Source: CAD feature listing. Evaluate the final solid. Frame: model axes, mm. Face numbers are marked on the shaded views. Give positions to 0.01 mm unless a question says otherwise; leave off trailing zeros. Order: outer loops, then holes, each group sorted by start corner. A loop starts at its lowest first (then second) coordinate and runs counter-clockwise, first axis right, second up.
1) Material intervals for line 1 (Z direction, x = 18.25, y = 0.6); line 2 (Z direction, x = 18.25, y = 3.2); line 3 (X direction, y = 1, z = 38.5), sorted ascending.
2) Draft query along X for the marked faces 1, 2 and 3. Return one class per face: released by +X, released by -X, zero draft, split by the parting line, or undercut.
3) First-contact query: P1, Ø4, axis at y = 10.5, z = -13.5, coming from the +X side; P2, Ø10, axis at y = 13.5, z = 25, coming from the -X side; P3, Ø11, axis at x = 41, y = 6.5, coming from the -Z side. Flat tips, straight axial feed; report the tip coordinate or a pass-through.
4) Section C-C, the plane x = 18.25. Return loops of the section in (y, z).
5) Section D-D, the plane z = 16.5. Return loops of the section in (x, y), plus the area to 3 significant figures.
6) Section B-B, the plane x = 0. Return loops of the section in (y, z).
7) Section A-A, the plane z = 0. Return loops of the section in (x, y), plus the area to 3 significant figures.
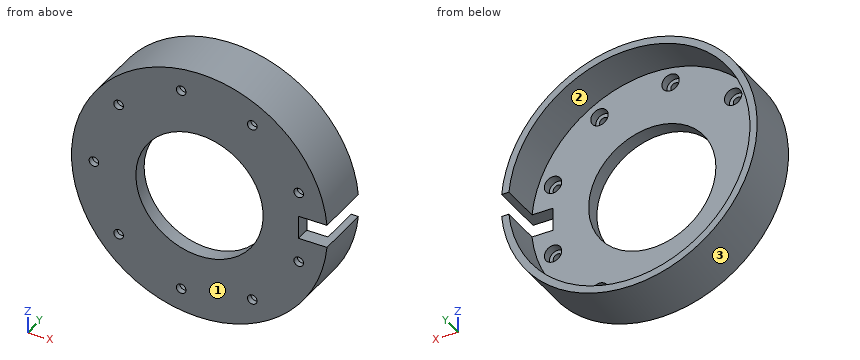
Autodesk Inventor part; units mm, degrees
ref_plane "YZ Plane" through (0, 0, 0) normal (1, 0, 0) x (0, 1, 0)
ref_plane "XZ Plane" through (0, 0, 0) normal (0, 1, 0) x (-1, 0, 0)
ref_plane "XY Plane" through (0, 0, 0) normal (0, 0, 1) x (1, 0, 0)
sketch "スケッチ1" plane through (0, 0, 0) normal (0, 1, 0) x (-1, 0, 0)
  circle A0 centre (0, 0) radius 44.25
  circle A1 centre (0, 0) radius 22
  dimension "d0" = 88.5
  dimension "d3" = 44
extrude "押し出し1" add sketch "スケッチ1" along normal blind 5
sketch "スケッチ2" plane through (0, 5, 0) normal (0, 1, 0) x (1, 0, 0)
  circle A0 centre (0, 0) radius 36.5
  point P0 (-36.5, 0)
  point P1 (-27.9606, -23.4617)
  point P2 (-6.3382, -35.9455)
  point P3 (18.25, -31.6099)
  point P4 (34.2988, -12.4837)
  point P5 (34.2988, 12.4837)
  point P6 (18.25, 31.6099)
  point P7 (-6.3382, 35.9455)
  point P8 (-27.9606, 23.4617)
  dimension "d4" = 73
  dimension "d7" = 360
hole "穴1" at (-36.5, 5, 0) at (-27.9606, 5, 23.4617) at (-6.3382, 5, 35.9455) at (18.25, 5, 31.6099) at (34.2988, 5, 12.4837) at (34.2988, 5, -12.4837) at (18.25, 5, -31.6099) at (-6.3382, 5, -35.9455) at (-27.9606, 5, -23.4617) direction (0, -1, 0) diameter 3.3 end through all
sketch "スケッチ3" plane through (0, 5, 0) normal (0, 1, 0) x (1, 0, 0)
  circle A0 centre (-36.5, 0) radius 1.65
  circle A1 centre (-36.5, 0) radius 3
  circle A2 centre (-27.9606, -23.4617) radius 3
  circle A3 centre (-6.3382, -35.9455) radius 3
  circle A4 centre (18.25, -31.6099) radius 3
  circle A5 centre (34.2988, -12.4837) radius 3
  circle A6 centre (34.2988, 12.4837) radius 3
  circle A7 centre (18.25, 31.6099) radius 3
  circle A8 centre (-6.3382, 35.9455) radius 3
  circle A9 centre (-27.9606, 23.4617) radius 3
  point P0 (0, 0)
  dimension "d16" = 6
  dimension "d19" = 360
extrude "押し出し2" cut sketch "スケッチ3" against normal blind 3 contours A0 | A1 | A2 | A3 | A4 | A5 | A6 | A7 | A8 | A9
sketch "スケッチ4" plane through (0, 5, 0) normal (0, 1, 0) x (1, 0, 0)
  circle A0 centre (0, 0) radius 41.75
  circle A1 centre (0, 0) radius 44.25
  line L0 (0, 0) -> (44.25, 0)
  line L1 (44.25, 0) -> (44.25, 4)
  line L2 (44.25, 4) -> (0, 4)
  line L3 (0, 4) -> (0, 0)
  line L4 (44.25, 0) -> (44.25, -4)
  line L5 (44.25, -4) -> (0, -4)
  line L6 (0, -4) -> (0, 0)
  point P0 (44.0688, -4)
  point P1 (41.5579, -4)
  point P2 (41.5579, 4)
  point P3 (44.0688, 4)
  dimension "d23" = 2.5
  dimension "d24" = 4
extrude "押し出し3" add sketch "スケッチ4" along normal blind 14 contours A0 L5 A1 L2
sketch "スケッチ6" plane through (0, 5, 0) normal (0, 1, 0) x (1, 0, 0)
  circle A0 centre (0, 0) radius 44.25
  line L0 (44.0688, 4) -> (41.5579, 4)
  line L1 (44.25, 0) -> (34.25, 0)
  line L2 (34.25, 0) -> (34.25, 4)
  line L3 (34.25, 4) -> (44.25, 4)
  line L4 (44.25, 4) -> (44.25, 0)
  line L5 (44.0688, -4) -> (29.25, -4)
  line L6 (34.25, 0) -> (34.25, -4)
  line L7 (44.25, -4) -> (44.25, 0)
  point P0 (29.25, 4)
  dimension "d31" = 10
extrude "押し出し5" cut sketch "スケッチ6" against normal blind 14 contours L1 L2 L3 L0 A0 | A0 L5 L6 L1
sketch "スケッチ7" plane through (0, 5, 0) normal (0, 1, 0) x (1, 0, 0)
  circle A0 centre (0, 0) radius 58
  arc A1 (41.5579, 4) -> (41.5579, -4) centre (0, 0) ccw
  circle A2 centre (0, 0) radius 22
  circle A3 centre (0, 0) radius 15
  circle A4 centre (40, 0) radius 18
  circle A5 centre (0, 0) radius 22
  circle A6 centre (0, 0) radius 22
  dimension "d36" = 30
  dimension "d37" = 7
  dimension "d39" = 36
  dimension "d41" = 116
properties part number "cablepart1"
From the geometry:
1. line 1: z = -40.31 to -33.26, -29.96 to -12.29, 12.29 to 29.96, 33.26 to 40.31
1. line 2: z = -40.31 to -34.61, -28.61 to -12.29, 12.29 to 28.61, 34.61 to 40.31
1. line 3: x = -21.81 to 21.81
2. face 1: zero draft
2. face 2: undercut
2. face 3: split by the parting line
3. P1: stops at x = 42.73
3. P2: stops at x = -39.47
3. P3: stops at z = -26.42
4. outline: (0, -40.31) - (19, -40.31) - (19, -37.55) - (5, -37.55) - (5, -34.61) - (2, -34.61) - (2, -33.26) - (0, -33.26) - close; (0, -29.96) - (2, -29.96) - (2, -28.61) - (5, -28.61) - (5, -12.29) - (0, -12.29) - close; (0, 12.29) - (5, 12.29) - (5, 28.61) - (2, 28.61) - (2, 29.96) - (0, 29.96) - close; (0, 33.26) - (2, 33.26) - (2, 34.61) - (5, 34.61) - (5, 37.55) - (19, 37.55) - (19, 40.31) - (0, 40.31) - close
5. outline: (-41.06, 0) - (-14.55, 0) - (-14.55, 5) - (-38.35, 5) - (-38.35, 19) - (-41.06, 19) - close; (14.55, 0) - (41.06, 0) - (41.06, 19) - (38.35, 19) - (38.35, 5) - (14.55, 5) - close
5. area: 341 mm2
6. outline: (0, -44.25) - (19, -44.25) - (19, -41.75) - (5, -41.75) - (5, -22) - (0, -22) - close; (0, 22) - (5, 22) - (5, 41.75) - (19, 41.75) - (19, 44.25) - (0, 44.25) - close
7. outline: (-44.25, 0) - (-38.15, 0) - (-38.15, 2) - (-39.5, 2) - (-39.5, 5) - (-41.75, 5) - (-41.75, 19) - (-44.25, 19) - close; (-34.85, 0) - (-22, 0) - (-22, 5) - (-33.5, 5) - (-33.5, 2) - (-34.85, 2) - close; (22, 0) - (34.25, 0) - (34.25, 5) - (22, 5) - close
7. area: 183 mm2
